```python
from build123d import *

# Parameters (mm, degrees)
F0_W     = 38.1
F0_H     = 31.75
F1_DEPTH = 25.4
F2_W     = 29.7038885713
F2_H     = 5.2352226339
F2_H_2   = 5.7432226181
F3_DEPTH = 31.751


with BuildPart() as f1:
    # F0 (on Front) → F1 (new body)
    with BuildSketch(Plane.XZ):
        with Locations((19.05, 15.875)):
            Rectangle(F0_W, F0_H)
    extrude(amount=F1_DEPTH)

    # F2 (on face) → F3 (cut, through all)
    with BuildSketch(Plane.XY.offset(31.75)):
        with Locations((23.2480557144, -2.617611317)):
            Rectangle(F2_W, F2_H)
        with Locations((23.2480557144, -22.5283886909)):
            Rectangle(F2_W, F2_H_2)
    extrude(amount=-F3_DEPTH, mode=Mode.SUBTRACT)


solid = f1.part
```
Could you check a few things on this model? Use its own coordinates, in mm. A direction names the side the tool comes from. Coordinates: 2 decimals unless noted, no trailing zeros. Write each loop counter-clockwise with the first axis right and the second up, starting at its lowest first coordinate (ties: lowest second). Pieces come first, ordered by that corner, then holes. Notation, with made-up numbers: (-28.5, 25) -> (-16.5, 25) arc R24 cw to (-16.5, 44) -> close; hole circle Ø3 at (11.5, 20.25). An arc over 180 degrees is marked (long way). Write item = value, one per line. Start each with the question number.
(1) I want a section at C-C (x = 29.5). Please give me the cut outline in (y, z), plus the area to 3 significant figures.
(2) I want a section at A-A (z = 28). Please give me the cut outline in (x, y).
(3) I need wall thicknesses on line 1 (X direction, y = -22.5, z = 26); line 2 (Y direction, x = 11.5, z = 13). Which ranges of each line are inside material? Lowest first, please. Write a range as [from, to].
(4) Which directions (+Z, -Z, +X, -X, +Y, -Y) give clear straight access to the entire face, cutting with the end or side of a thin tool? Please do faces 1 (the face through (15, -13, 31.75)), 2 (the face through (8.396, -23, 16)), 3 (the face through (23, -5.235, 16)).
(5) I want a section at B-B (y = -2). Please give me the cut outline in (x, z), plus the area to 3 significant figures.
(6) Will these pins go through, and if not, where does the flat tip stop? pin 1 (6 mm diameter, centred on x = 32, y = -20, fed in from +Z); pin 2 (4 mm diameter, centred on x = 20, z = 16.5, fed in from +Y); pin 3 (2.5 mm diameter, centred on y = -2.5, z = 14, fed in from +X).
Result set:
q1.outline = (-19.66, 0) -> (-5.24, 0) -> (-5.24, 31.75) -> (-19.66, 31.75) -> close
q1.area = 458 mm2
q2.outline = (0, -25.4) -> (8.4, -25.4) -> (8.4, -19.66) -> (38.1, -19.66) -> (38.1, -5.24) -> (8.4, -5.24) -> (8.4, 0) -> (0, 0) -> close
q3.line_1 = [0, 8.4]
q3.line_2 = [-19.66, -5.24]
q4.face_1 = +Z, +X, -X, +Y, -Y
q4.face_2 = +Z, -Z, +X, -Y
q4.face_3 = +Z, -Z, +X, +Y
q5.outline = (0, 0) -> (8.4, 0) -> (8.4, 31.75) -> (0, 31.75) -> close
q5.area = 267 mm2
q6.pin_1 = 31.75
q6.pin_2 = -5.24
q6.pin_3 = 8.4
